Check sheet for the drawn part. Datum: minimum x, y, z corner. Units: mm. Coordinates: 2 decimals unless noted, no trailing zeros. Write each loop counter-clockwise with the first axis right and the second up, starting at its lowest first coordinate (ties: lowest second). Pieces come first, ordered by that corner, then holes. Notation, with made-up numbers: (-31.75, -36.75) -> (3.25, -36.75) arc R20 cw to (3.25, -18.75) -> close; hole circle Ø7 at (77.25, -15). An arc over 180 degrees is marked (long way). Answer in a Markdown table with one row per item. Add a question column.
1. Cross-section at A-A on y = 1.25. Record the cut outline in (x, z), and give its area (3 significant figures).
2. Cross-section at C-C on z = 184.15. Record the cut outline in (x, y).
3. Depth check by flat-ended pin: P1, Ø1.9, axis at x = 125, y = 1.5, coming from the -Z side; P2, Ø2, axis at x = 50, y = 3.5, coming from the -Z side; P3, Ø1.5, axis at y = 1.5, z = 21.5, coming from the -X side. Enter the tip coordinate at first touch or a pass-through.
4. Cross-section at B-B on x = 63.5. Record the cut outline in (y, z).
5. Scan lines: L1, parallel to Z at x = 63.5, y = 5; L2, parallel to X at y = 4.75, z = 89; L3, parallel to X at y = 3.5, z = 105. Record each from-to range of solid material in increasing order. Write a range as from..to.
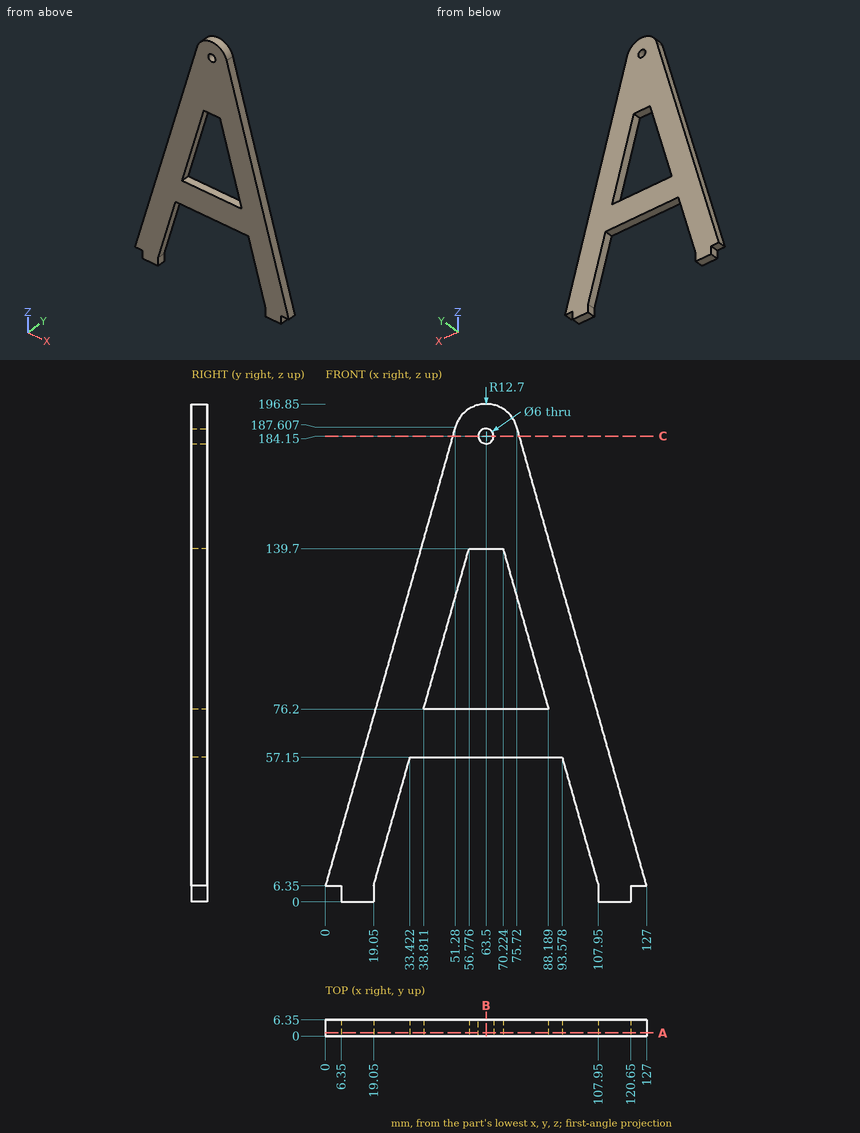
Results found:
| question | item | result |
|---|---|---|
| 1 | outline | (0, 6.35) -> (6.35, 6.35) -> (6.35, 0) -> (19.05, 0) -> (19.05, 6.35) -> (33.42, 57.15) -> (93.58, 57.15) -> (107.95, 6.35) -> (107.95, 0) -> (120.65, 0) -> (120.65, 6.35) -> (127, 6.35) -> (75.72, 187.61) arc R12.7 ccw to (51.28, 187.61) -> close; hole (38.81, 76.2) -> (88.19, 76.2) -> (70.22, 139.7) -> (56.78, 139.7) -> close; hole circle Ø6 at (63.5, 184.15) |
| 1 | area | 8,240 mm^2 |
| 2 | outline | (50.3, 0) -> (60.5, 0) -> (60.5, 6.35) -> (50.3, 6.35) -> close; (66.5, 0) -> (76.7, 0) -> (76.7, 6.35) -> (66.5, 6.35) -> close |
| 3 | P1 | stops at z = 6.35 |
| 3 | P2 | stops at z = 57.15 |
| 3 | P3 | stops at x = 4.07 |
| 4 | outline | (0, 57.15) -> (6.35, 57.15) -> (6.35, 76.2) -> (0, 76.2) -> close; (0, 139.7) -> (6.35, 139.7) -> (6.35, 181.15) -> (0, 181.15) -> close; (0, 187.15) -> (6.35, 187.15) -> (6.35, 196.85) -> (0, 196.85) -> close |
| 5 | L1 | z = 57.15..76.2, 139.7..181.15, 187.15..196.85 |
| 5 | L2 | x = 23.38..42.43, 84.57..103.62 |
| 5 | L3 | x = 27.91..46.96, 80.04..99.09 |
